```python
from build123d import *

# Parameters (mm, degrees)
SKETCH1_W           = 70
SKETCH1_H           = 5
BOSS_EXTRUDE1_DEPTH = 30
SKETCH4_W           = 70
SKETCH4_H           = 15
BOSS_EXTRUDE2_DEPTH = 10
SKETCH5_W           = 4
SKETCH5_H           = 10
CUT_EXTRUDE1_DEPTH  = 10
SKETCH6_W           = 4
SKETCH6_H           = 10
CUT_EXTRUDE2_DEPTH  = 10
SKETCH7_W           = 4
SKETCH7_H           = 10
CUT_EXTRUDE3_DEPTH  = 10
SKETCH8_W           = 4
SKETCH8_H           = 10
CUT_EXTRUDE4_DEPTH  = 10
FILLET5_R           = 1


with BuildPart() as part:
    # Sketch1 → Boss-Extrude1 (new body)
    with BuildSketch(Plane(origin=(0, 0, 0), x_dir=(1, 0, 0), z_dir=(0, 1, 0))):
        with Locations((35, 2.5)):
            Rectangle(SKETCH1_W, SKETCH1_H)
    extrude(amount=BOSS_EXTRUDE1_DEPTH)

    # Sketch4 → Boss-Extrude2 (add)
    with BuildSketch(Plane(origin=(0, 0, 0), x_dir=(-1, 0, 0), z_dir=(0, -1, 0))):
        with Locations((-35, 12.5)):
            Rectangle(SKETCH4_W, SKETCH4_H)
    extrude(amount=-BOSS_EXTRUDE2_DEPTH)

    # Sketch5 → Cut-Extrude1 (cut)
    with BuildSketch(Plane(origin=(0, 10, 0), x_dir=(1, 0, 0), z_dir=(0, 1, 0))):
        with Locations((17, 15)):
            Rectangle(SKETCH5_W, SKETCH5_H)
    extrude(amount=-CUT_EXTRUDE1_DEPTH, mode=Mode.SUBTRACT)

    # Sketch6 → Cut-Extrude2 (cut)
    with BuildSketch(Plane(origin=(0, 10, 0), x_dir=(1, 0, 0), z_dir=(0, 1, 0))):
        with Locations((29, 15)):
            Rectangle(SKETCH6_W, SKETCH6_H)
    extrude(amount=-CUT_EXTRUDE2_DEPTH, mode=Mode.SUBTRACT)

    # Sketch7 → Cut-Extrude3 (cut)
    with BuildSketch(Plane(origin=(0, 10, 0), x_dir=(1, 0, 0), z_dir=(0, 1, 0))):
        with Locations((41, 15)):
            Rectangle(SKETCH7_W, SKETCH7_H)
    extrude(amount=-CUT_EXTRUDE3_DEPTH, mode=Mode.SUBTRACT)

    # Sketch8 → Cut-Extrude4 (cut)
    with BuildSketch(Plane(origin=(0, 10, 0), x_dir=(1, 0, 0), z_dir=(0, 1, 0))):
        with Locations((53, 15)):
            Rectangle(SKETCH8_W, SKETCH8_H)
    extrude(amount=-CUT_EXTRUDE4_DEPTH, mode=Mode.SUBTRACT)

    # Fillet5
    fillet5_edges = [part.edges().sort_by_distance(p)[0] for p in [
        (70, 30, -2.5),
        (35, 30, -5),
        (62.5, 0, -20),
        (70, 5, -20),
        (0, 10, -12.5),
        (0, 5, -20),
        (35, 10, -5),
        (70, 10, -12.5),
        (62.5, 10, -20),
        (7.5, 10, -20),
        (7.5, 0, -20),
        (15, 5, -20),
        (19, 10, -15),
        (19, 5, -20),
        (17, 0, -10),
        (15, 0, -15),
        (19, 0, -15),
        (15, 10, -15),
        (17, 10, -10),
        (0, 30, -2.5),
        (23, 10, -20),
        (23, 0, -20),
        (27, 0, -15),
        (27, 5, -20),
        (31, 0, -15),
        (31, 5, -20),
        (29, 0, -10),
        (27, 10, -15),
        (29, 10, -10),
        (31, 10, -15),
        (70, 0, -10),
        (35, 0, 0),
        (0, 0, -10),
        (35, 10, -20),
        (35, 0, -20),
        (39, 0, -15),
        (39, 5, -20),
        (43, 0, -15),
        (43, 5, -20),
        (41, 0, -10),
        (39, 10, -15),
        (41, 10, -10),
        (43, 10, -15),
        (35, 30, 0),
        (47, 10, -20),
        (0, 20, -5),
        (47, 0, -20),
        (70, 20, -5),
        (70, 15, 0),
        (0, 15, 0),
        (51, 0, -15),
        (51, 5, -20),
        (55, 0, -15),
        (55, 5, -20),
        (53, 0, -10),
        (51, 10, -15),
        (53, 10, -10),
        (55, 10, -15),
    ]]
    fillet(fillet5_edges, radius=FILLET5_R)


solid = part.part
```
CAD build for the part. Positions are in the model's coordinates, mm. A direction names the side the tool comes from. Round coordinates to 2 decimals unless told otherwise and drop trailing zeros. Write each loop counter-clockwise with the first axis right and the second up, starting at its lowest first coordinate (ties: lowest second). Pieces come first, ordered by that corner, then holes. Notation, with made-up numbers: (18.5, 70.25) - (70.5, 70.25) arc R15 cw to (70.5, 93.25) - close; hole circle Ø1 at (12.25, 53.5). An arc over 180 degrees is marked (long way). Return JSON: item names as keys, results as strings. Group by question number.
Item 1: 3-axis set-ups, long thin cutter, end or side, ignore diameter. For faces 4 (the face through (35, 20, -5)), 5 (the face through (17, 5, -10)), 6 (the face through (8, 5, -20)): which of +Z, -Z, +X, -X, +Y, -Y reach the whole face in a straight line?
Item 2: Probe probe 1 along X at (y, z) = (9, -11.25); probe 2 along Z at (x, y) = (35.5, 11.25); probe 3 along Y at (x, z) = (32.5, -17.25). List the from-to ranges inside material, lowest first.
Item 3: Band-saw the part on D-D on z = -7.75. List the corners of the cut face in (x, y), plus the area to 3 significant figures.
Item 4: Band-saw the part on C-C on z = -13. State how many separate pieces and enclosed holes the cut face has, plus the area to 3 significant figures.
Item 5: Flat gauge pins, fed straight in: pin 1 Ø10 at (y, z) = (11, -16.5) entering from -X; pin 2 Ø1.2 at (x, y) = (29.5, 4.5) entering from -Z; pin 3 Ø6.5 at (x, z) = (32, -15) entering from +Y; pin 4 Ø5.5 at (x, y) = (32, 17) entering from -Z. Where does each tip first touch, or does it go through?
Item 6: Mould opens along X. For faces 1 (the face through (0, 8.6, -7.9)), 2 (the face through (35, 0, -10)), 3 (the face through (29, 5, -10)) say: +X half, -X half, draft (parallel to the pull), parting line (faces both ways), or undercut.
Item 7: Band-saw the part on B-B on x = 24. List the corners of the cut face in (y, z).
Item 8: Band-saw the part on A-A on y = 22.25. List the corners of the cut face in (x, z), plus the area to 3 significant figures.
Resolved:
{
 "1": {"face 4": "-Z, +X, -X, +Y", "face 5": "-Z, +Y, -Y", "face 6": "-Z, +X, -X, +Y, -Y"},
 "2": {"probe 1": "x = 0 to 15, 19 to 27, 31 to 39, 43 to 51, 55 to 70", "probe 2": "z = -5 to 0", "probe 3": "y = 0 to 10"},
 "3": {"outline": "(0, 1) arc R1 ccw to (1, 0) - (69, 0) arc R1 ccw to (70, 1) - (70, 9) arc R1 ccw to (69, 10) - (1, 10) arc R1 ccw to (0, 9) - close", "area": "699 mm²"},
 "4": {"separate pieces": "5", "enclosed holes": "0", "area": "536 mm²"},
 "5": {"pin 1": "stops at x = 0", "pin 2": "stops at z = -10", "pin 3": "stops at y = 10", "pin 4": "stops at z = -5"},
 "6": {"face 1": "-X half", "face 2": "draft", "face 3": "undercut"},
 "7": {"outline": "(0, -19) arc R1 ccw to (1, -20) - (9, -20) arc R1 ccw to (10, -19) - (10, -6) arc R1 cw to (11, -5) - (29, -5) arc R1 ccw to (30, -4) - (30, -1) arc R1 ccw to (29, 0) - (1, 0) arc R1 ccw to (0, -1) - close"},
 "8": {"outline": "(0, -4) arc R1 ccw to (1, -5) - (69, -5) arc R1 ccw to (70, -4) - (70, -1) arc R1 ccw to (69, 0) - (1, 0) arc R1 ccw to (0, -1) - close", "area": "349 mm²"}
}
